Check sheet for the modelled part. Datum: model origin and axes. Units: mm. Face numbers are marked on the shaded views. A direction names the side the tool comes from. Round coordinates to 2 decimals unless told otherwise and drop trailing zeros. Loops run counter-clockwise (first coordinate to the right, second up) from the corner with the lowest first, then second, coordinate; pieces in that order, holes last. Notation, with made-up numbers: (-33.5, 16) - (-0.5, 16) arc R13 cw to (-0.5, 41) - close; hole circle Ø2 at (70, 45). An arc over 180 degrees is marked (long way). Return JSON: item names as keys, results as strings.
from build123d import *

# Parameters (mm, degrees)
SKETCH1_R             = 3
BOSS_EXTRUDE1_DEPTH   = 8
SKETCH1_3_R           = 2
BOSS_EXTRUDE2_DEPTH   = 5
FILLET1_R             = 2
M3_TAPPED_HOLE1_D     = 3
M3_TAPPED_HOLE1_DEPTH = 8.5
M3_TAPPED_HOLE1_TIP   = 0.901290929


with BuildPart() as part:
    # Sketch1 → Boss-Extrude1 (new body)
    with BuildSketch(Plane(origin=(0, 0, 0), x_dir=(1, 0, 0), z_dir=(0, 1, 0))):
        with BuildLine():
            ThreePointArc((6, 0), (0, 6), (-6, 0))
            Line((-6, 0), (-5.815384615, -1.476923077))
            ThreePointArc((-5.815384615, -1.476923077), (0, -6), (5.815384615, -1.476923077))
            Line((5.815384615, -1.476923077), (6, 0))
        make_face()
        Circle(SKETCH1_R, mode=Mode.SUBTRACT)
    extrude(amount=BOSS_EXTRUDE1_DEPTH)

    # Sketch1<3> → Boss-Extrude2 (add)
    with BuildSketch(Plane(origin=(0, 0, 0), x_dir=(1, 0, 0), z_dir=(0, 1, 0))):
        with BuildLine():
            ThreePointArc((5.815384615, -1.476923077), (0, -6), (-5.815384615, -1.476923077))
            Line((-5.815384615, -1.476923077), (-4, -16))
            ThreePointArc((-4, -16), (0, -20), (4, -16))
            Line((4, -16), (5.815384615, -1.476923077))
        make_face()
        with Locations((0, -16)):
            Circle(SKETCH1_3_R, mode=Mode.SUBTRACT)
    extrude(amount=BOSS_EXTRUDE2_DEPTH)

    # Fillet1
    fillet1_edges = [part.edges().sort_by_distance(p)[0] for p in [
        (0, 5, 6),
    ]]
    fillet(fillet1_edges, radius=FILLET1_R)

    # M3 Tapped Hole1
    with Locations(Plane(origin=(0, 0, -8), x_dir=(1, 0, 0), z_dir=(0, 0, -1))):
        with Locations((0, -5)):
            Hole(M3_TAPPED_HOLE1_D / 2, depth=M3_TAPPED_HOLE1_DEPTH)
            with Locations((0, 0, -(M3_TAPPED_HOLE1_DEPTH + M3_TAPPED_HOLE1_TIP / 2))):  # 118° drill point
                Cone(0, M3_TAPPED_HOLE1_D / 2, M3_TAPPED_HOLE1_TIP, mode=Mode.SUBTRACT)


solid = part.part
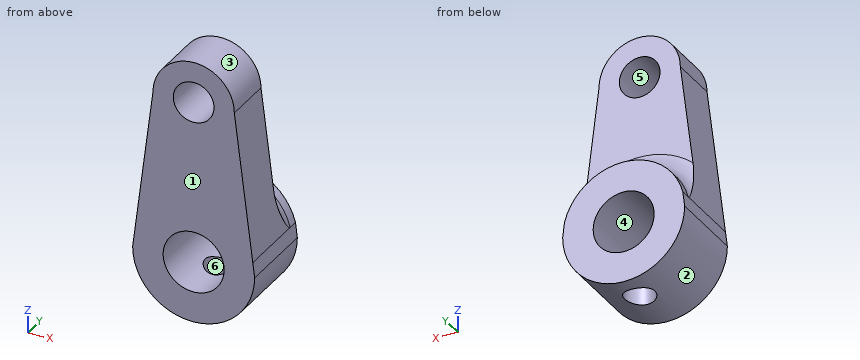
Q1. Sectioned sample at C-C (z = 17). Enter the section's corners in (x, y), plus the area to 3 significant figures.
Answer key:
{"outline": "(-3.87, 0) - (-1.73, 0) - (-1.73, 5) - (-3.87, 5) - close; (1.73, 0) - (3.87, 0) - (3.87, 5) - (1.73, 5) - close", "area": "21.4 mm²"}
Q2. Scan lines: probe 1 along Z at (x, y) = (0, 2.95); probe 2 along Z at (x, y) = (0.75, 0.75); probe 3 along Z at (x, y) = (0, 4.75). Record each from-to range of solid material in increasing order. Write a range as [from, to].
Answer key:
{"probe 1": "z = [-6, -3], [3, 14], [18, 20]", "probe 2": "z = [-5.95, -2.9], [2.9, 14.15], [17.85, 19.93]", "probe 3": "z = [3, 14], [18, 20]"}
Q3. Sectioned sample at B-B (y = 6.75). Enter the section's corners in (x, z).
Answer key:
{"outline": "(-6, 0) arc R6 ccw to (6, 0) - (5.8, 1.59) arc R6.02 ccw to (-5.8, 1.59) - close; hole circle Ø6 at (0, 0)"}
Q4. Draft check along Z on the marked faces 1, 2, 3 and 4. Enter one of: released by +Z, released by -Z, zero draft, split by the parting line, or undercut.
Answer key:
{"face 1": "zero draft", "face 2": "released by -Z", "face 3": "released by +Z", "face 4": "undercut"}
Q5. Sectioned sample at D-D (y = 5.25). Enter the section's corners in (x, z).
Answer key:
{"outline": "(-6, 0) arc R6 ccw to (-1.48, -5.81) - (-1.48, -2.61) arc R3 cw (long way) to (1.48, -2.61) - (1.48, -5.81) arc R6 ccw to (6, 0) - (5.44, 4.45) arc R7.03 ccw to (-5.44, 4.45) - close"}
Q6. Tool access check on the marked faces 5 and 6. Record the directions out of +Z, -Z, +X, -X, +Y, -Y that give a thin tool (end or side, any length) a straight path to the whole face; none if there is none.
Answer key:
{"face 5": "+Y, -Y", "face 6": "-Z"}
Q7. Sectioned sample at A-A (x = 0). Enter the section's corners in (y, z), plus the area to 3 significant figures.
Answer key:
{"outline": "(0, -6) - (3.5, -6) - (3.5, -3) - (0, -3) - close; (0, 3) - (8, 3) - (8, 6) - (7, 6) arc R2 cw to (5, 8) - (5, 14) - (0, 14) - close; (0, 18) - (5, 18) - (5, 20) - (0, 20) - close; (6.5, -6) - (8, -6) - (8, -3) - (6.5, -3) - close", "area": "89.9 mm²"}
Q8. Depth check by flat-ended pin: P1, Ø4, axis at x = -1, y = 3, coming from the +Z side; P2, Ø1.5, axis at x = -4, y = 6, coming from the +Z side; P3, Ø1.5, axis at y = 4.5, z = -1.5, coming from the +X side; P4, Ø1, axis at y = 4, z = 11.5, coming from the +X side (3 decimals). Enter the tip coordinate at first touch or a pass-through.
Answer key:
{"P1": "stops at z = 20", "P2": "stops at z = 5.86", "P3": "stops at x = 5.95", "P4": "stops at x = 4.625"}
